```python
from build123d import *

# Parameters (mm, degrees)
F1_DEPTH = 25.4
F2_SIZE  = 5.08
F3_R     = 15.2778949267
F5_DEPTH = 25


with BuildPart() as f1:
    # F0 (on Front) → F1 (new body)
    with BuildSketch(Plane.XZ):
        with BuildLine():
            Line((50.8587062359, 342.0623540878), (-50.8587062359, 342.0623540878))
            Line((-50.8587062359, 342.0623540878), (-50.8587062359, -342.0623540878))
            Line((-50.8587062359, -342.0623540878), (0.0587062359, -342.0623540878))
            ThreePointArc((0.0587062359, -342.0623540878), (35.9797307202, -327.1833785721), (50.8587062359, -291.2623540878))
            Line((50.8587062359, -291.2623540878), (50.8587062359, 342.0623540878))
        make_face()
    extrude(amount=F1_DEPTH)

    # F2
    f2_edges = [f1.edges().sort_by_distance(p)[0] for p in [
        (-50.858706, -12.7, 342.062354),
    ]]
    chamfer(f2_edges, length=F2_SIZE)

    # F3
    f3_edges = [f1.edges().sort_by_distance(p)[0] for p in [
        (50.858706, -12.7, 342.062354),
    ]]
    fillet(f3_edges, radius=F3_R)

    # F4 (on face) → F5 (join)
    with BuildSketch(Plane(origin=(0, 0, 0), x_dir=(-1, 0, 0), z_dir=(0, 1, 0))):
        with BuildLine():
            ThreePointArc((27.986776288, -327.9091639399), (109.1739171381, -356.6419759562), (160.3966848346, -287.4093651772))
            ThreePointArc((160.3966848346, -287.4093651772), (145.5285553941, -243.4570500067), (107.0309394681, -217.5572266497))
            ThreePointArc((107.0309394681, -217.5572266497), (107.3433284277, -222.2019166399), (107.4475276889, -226.8559336662))
            ThreePointArc((107.4475276889, -226.8559336662), (85.2031326925, -291.1322247111), (27.986776288, -327.9091639399))
        make_face()
        with BuildLine():
            ThreePointArc((107.4475276889, -226.8559336662), (107.3433284277, -222.2019166399), (107.0309394681, -217.5572266497))
            ThreePointArc((107.0309394681, -217.5572266497), (29.1405817858, -245.2503223082), (27.986776288, -327.9091639399))
            ThreePointArc((27.986776288, -327.9091639399), (85.2031326925, -291.1322247111), (107.4475276889, -226.8559336662))
        make_face()
        with BuildLine():
            ThreePointArc((27.986776288, -327.9091639399), (29.1405817858, -245.2503223082), (107.0309394681, -217.5572266497))
            ThreePointArc((107.0309394681, -217.5572266497), (-81.0768529773, -166.3025021553), (27.986776288, -327.9091639399))
        make_face()
    extrude(amount=F5_DEPTH)


solid = f1.part
```
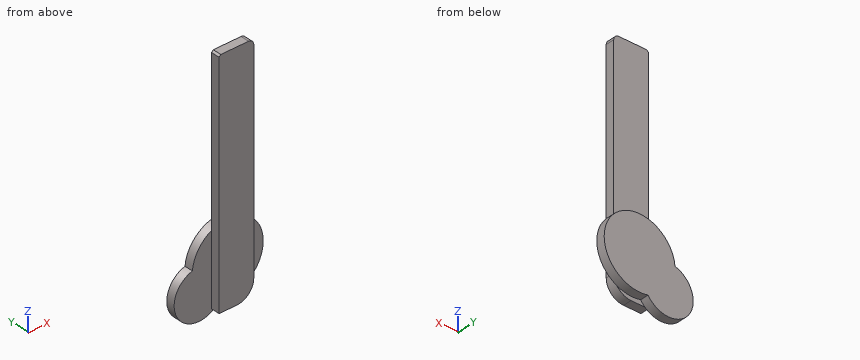
Input: part model. Units: mm. Frame: model coordinates. Give positions to 0.01 mm unless a question says otherwise; leave off trailing zeros. Order: outer loops, then holes, each group sorted by start corner. A loop starts at its lowest first (then second) coordinate and runs counter-clockwise, first axis right, second up.
1. Pin query (flat end, axial travel): pin 1 Ø6 at (x, y) = (-19, -6.5) entering from -Z; pin 2 Ø5 at (x, y) = (-38.5, 19) entering from +Z; pin 3 Ø12.5 at (y, z) = (-7, 153.5) entering from -X. Return the tip coordinate at first contact, or that it passes through.
Computed:
pin 1: stops at z = -342.06
pin 2: stops at z = -128.09
pin 3: stops at x = -50.86
2. Cut plane D-D (x = -114). Return loops of the section in (y, z), and give its area (3 significant figures).
Computed:
outline: (0, -354.98) - (25, -354.98) - (25, -219.84) - (0, -219.84) - close
area: 3,380 mm2
3. Cut plane B-B (z = 168). Return loops of the section in (x, y), and give its area (3 significant figures).
Computed:
outline: (-50.86, -25.4) - (50.86, -25.4) - (50.86, 0) - (-50.86, 0) - close
area: 2,580 mm2
4. Line query: probe 1 along X at (y, z) = (-1.5, -145); probe 2 along Y at (x, z) = (42, 29.5); probe 3 along Z at (x, y) = (-35.5, -2.5). Output: solid intervals per line, ascending.
Computed:
probe 1: x = -50.86 to 50.86
probe 2: y = -25.4 to 0
probe 3: z = -342.06 to 342.06
5. Cut plane C-C (x = -7). Return loops of the section in (y, z).
Computed:
outline: (-25.4, -342.06) - (0, -342.06) - (0, -330.78) - (25, -330.78) - (25, -122.93) - (0, -122.93) - (0, 342.06) - (-25.4, 342.06) - close
6. Cut plane A-A (y = -9.5). Return loops of the section in (x, z).
Computed:
outline: (-50.86, -342.06) - (0.06, -342.06) arc R50.8 ccw to (50.86, -291.26) - (50.86, 326.78) arc R15.28 ccw to (35.58, 342.06) - (-45.78, 342.06) - (-50.86, 336.98) - close
